from build123d import *

# Parameters (mm, degrees)
SKETCH2_R                      = 22.5
SKETCH2_R_2                    = 14.5
USB_CHARGE_DEVICE_RING_DEPTH   = 10
RING_START                     = 70.540362552
RING_COMPLETION_DEPTH          = 10
SKETCH4_W                      = 45
SKETCH4_H                      = 23.80144284
LINK_TO_UNIT_CHASSIS_DEPTH     = 8
SKETCH5_W                      = 100
SKETCH5_H                      = 166
SKETCH5_W_2                    = 94
SKETCH5_H_2                    = 160
CHASSIS_WALLS_DEPTH            = 55
SKETCH6_W                      = 19
SKETCH6_H                      = 19
SKETCH6_R                      = 1.75
DISPLAY_FRAME_MOUNT_TABS_DEPTH = 3
SKETCH7_W                      = 94
SKETCH7_H                      = 68
SKETCH7_R                      = 1
RPI_MOUNT_SURFACE_DEPTH        = 3
SKETCH8_R                      = 3
SKETCH8_R_2                    = 1
RPI_MOUNT_BOSSES_DEPTH         = 2
F_50MM_FAN_HOLES_REACH         = 246.023
SKETCH9_R                      = 1.75
SKETCH9_R_2                    = 25
RJ45_CUTOUT_REACH              = 246.023
SKETCH10_R                     = 1.75
SKETCH10_W                     = 14
SKETCH10_H                     = 17


# Read off the part's stored shape, not the designer's step: RING COMPLETION
with BuildPart() as part:
    # Sketch2 → USB CHARGE DEVICE RING (new body)
    with BuildSketch(Plane(origin=(0, 40.270181276, 69.75), x_dir=(1, 0, 0), z_dir=(0, 0.500000000000001, 0.866025403784438))):
        with Locations(Location((0, -117.602885683, 0), (0, 0, 270))):
            Circle(SKETCH2_R)
        with Locations(Location((0, -117.602885683, 0), (0, 0, 270))):
            Circle(SKETCH2_R_2, mode=Mode.SUBTRACT)
    extrude(amount=-USB_CHARGE_DEVICE_RING_DEPTH)

    # RING COMPLETION outline → RING COMPLETION (add)
    with BuildSketch(Plane(origin=(0, 0, 0), x_dir=(1, 0, 0), z_dir=(0, 0.500000000000001, 0.866025403784438)).offset(RING_START)):
        with BuildLine():
            Line((-22.5, -68.102885683), (-22.5, -117.602885683))
            ThreePointArc((-22.5, -117.602885683), (0, -95.102885683), (22.5, -117.602885683))
            Line((22.5, -117.602885683), (22.5, -68.102885683))
            Line((22.5, -68.102885683), (-22.5, -68.102885683))
        make_face()
    extrude(amount=RING_COMPLETION_DEPTH)

    # Sketch4 → LINK TO UNIT CHASSIS (add)
    with BuildSketch(Plane(origin=(0, -18.708647797, 0), x_dir=(1, 0, 0), z_dir=(0, 1, 0))):
        with Locations((0, -91.900721421)):
            Rectangle(SKETCH4_W, SKETCH4_H)
    extrude(amount=-LINK_TO_UNIT_CHASSIS_DEPTH)

    # Sketch5 → CHASSIS WALLS (add)
    with BuildSketch(Plane(origin=(0, -13.208647797, 0), x_dir=(-1, 0, 0), z_dir=(0, -1, 0))):
        Rectangle(SKETCH5_W, SKETCH5_H)
        Rectangle(SKETCH5_W_2, SKETCH5_H_2, mode=Mode.SUBTRACT)
    extrude(amount=CHASSIS_WALLS_DEPTH)

    # Sketch6 → DISPLAY FRAME MOUNT TABS (add)
    # profile 1 of 3: a face of its own
    with BuildSketch(Plane(origin=(0, -13.208647797, 0), x_dir=(1, 0, 0), z_dir=(0, 1, 0))):
        with Locations((-40.5, -73.5)):
            Rectangle(SKETCH6_W, SKETCH6_H)
        with Locations(Location((-36, -69, 0), (0, 0, 270))):
            Circle(SKETCH6_R, mode=Mode.SUBTRACT)
    # profile 2 of 3: a face of its own
    with BuildSketch(Plane(origin=(0, -13.208647797, 0), x_dir=(1, 0, 0), z_dir=(0, 1, 0))):
        with Locations((40.5, -73.5)):
            Rectangle(SKETCH6_W, SKETCH6_H)
        with Locations(Location((36, -69, 0), (0, 0, 270))):
            Circle(SKETCH6_R, mode=Mode.SUBTRACT)
    # profile 3 of 3: a face of its own
    with BuildSketch(Plane(origin=(0, -13.208647797, 0), x_dir=(1, 0, 0), z_dir=(0, 1, 0))):
        with Locations((40.5, 73.5)):
            Rectangle(SKETCH6_W, SKETCH6_H)
        with Locations(Location((36, 69, 0), (0, 0, 270))):
            Circle(SKETCH6_R, mode=Mode.SUBTRACT)
    extrude(amount=-DISPLAY_FRAME_MOUNT_TABS_DEPTH)

    # Sketch7 → RPI MOUNT SURFACE (add)
    with BuildSketch(Plane(origin=(0, -32.208647797, 0), x_dir=(-1, 0, 0), z_dir=(0, -1, 0))):
        with Locations((0, -30.000000001)):
            Rectangle(SKETCH7_W, SKETCH7_H)
        with Locations(Location((7, -1.000000001, 0), (0, 0, 90))):
            Circle(SKETCH7_R, mode=Mode.SUBTRACT)
        with Locations(Location((-42, -1.000000001, 0), (0, 0, 90))):
            Circle(SKETCH7_R, mode=Mode.SUBTRACT)
        with Locations(Location((7, -59.000000001, 0), (0, 0, 90))):
            Circle(SKETCH7_R, mode=Mode.SUBTRACT)
        with Locations(Location((-42, -59.000000001, 0), (0, 0, 90))):
            Circle(SKETCH7_R, mode=Mode.SUBTRACT)
    extrude(amount=RPI_MOUNT_SURFACE_DEPTH)

    # Sketch8 → RPI MOUNT BOSSES (add)
    # profile 1 of 4: a face of its own
    with BuildSketch(Plane.XZ.offset(35.208647797)):
        with Locations(Location((42, 59.000000001, 0), (0, 0, 270))):
            Circle(SKETCH8_R)
        with Locations(Location((42, 59.000000001, 0), (0, 0, 270))):
            Circle(SKETCH8_R_2, mode=Mode.SUBTRACT)
    # profile 2 of 4: a face of its own
    with BuildSketch(Plane.XZ.offset(35.208647797)):
        with Locations(Location((42, 1.000000001, 0), (0, 0, 270))):
            Circle(SKETCH8_R)
        with Locations(Location((42, 1.000000001, 0), (0, 0, 270))):
            Circle(SKETCH8_R_2, mode=Mode.SUBTRACT)
    # profile 3 of 4: a face of its own
    with BuildSketch(Plane.XZ.offset(35.208647797)):
        with Locations(Location((-7, 1.000000001, 0), (0, 0, 270))):
            Circle(SKETCH8_R)
        with Locations(Location((-7, 1.000000001, 0), (0, 0, 270))):
            Circle(SKETCH8_R_2, mode=Mode.SUBTRACT)
    # profile 4 of 4: a face of its own
    with BuildSketch(Plane.XZ.offset(35.208647797)):
        with Locations(Location((-7, 59.000000001, 0), (0, 0, 270))):
            Circle(SKETCH8_R)
        with Locations(Location((-7, 59.000000001, 0), (0, 0, 270))):
            Circle(SKETCH8_R_2, mode=Mode.SUBTRACT)
    extrude(amount=RPI_MOUNT_BOSSES_DEPTH)

    # Sketch9 → 50MM FAN HOLES (cut, up to next)
    with BuildSketch(Plane(origin=(0, 0, -83), x_dir=(-1, 0, 0), z_dir=(0, 0, -1)), mode=Mode.PRIVATE) as f_50mm_fan_holes_sk1:
        with Locations((-23, -20.708647797)):
            Circle(SKETCH9_R)
    f_50mm_fan_holes_tool1 = extrude(f_50mm_fan_holes_sk1.sketch, amount=-F_50MM_FAN_HOLES_REACH, mode=Mode.PRIVATE) & part.part
    # Sketch9 → 50MM FAN HOLES (cut, up to next)
    with BuildSketch(Plane(origin=(0, 0, -83), x_dir=(-1, 0, 0), z_dir=(0, 0, -1)), mode=Mode.PRIVATE) as f_50mm_fan_holes_sk2:
        with Locations((17, -20.708647797)):
            Circle(SKETCH9_R)
    f_50mm_fan_holes_tool2 = extrude(f_50mm_fan_holes_sk2.sketch, amount=-F_50MM_FAN_HOLES_REACH, mode=Mode.PRIVATE) & part.part
    # Sketch9 → 50MM FAN HOLES (cut, up to next)
    with BuildSketch(Plane(origin=(0, 0, -83), x_dir=(-1, 0, 0), z_dir=(0, 0, -1)), mode=Mode.PRIVATE) as f_50mm_fan_holes_sk3:
        with Locations((17, -60.708647797)):
            Circle(SKETCH9_R)
    f_50mm_fan_holes_tool3 = extrude(f_50mm_fan_holes_sk3.sketch, amount=-F_50MM_FAN_HOLES_REACH, mode=Mode.PRIVATE) & part.part
    # Sketch9 → 50MM FAN HOLES (cut, up to next)
    with BuildSketch(Plane(origin=(0, 0, -83), x_dir=(-1, 0, 0), z_dir=(0, 0, -1)), mode=Mode.PRIVATE) as f_50mm_fan_holes_sk4:
        with Locations((-23, -60.708647797)):
            Circle(SKETCH9_R)
    f_50mm_fan_holes_tool4 = extrude(f_50mm_fan_holes_sk4.sketch, amount=-F_50MM_FAN_HOLES_REACH, mode=Mode.PRIVATE) & part.part
    # Sketch9 → 50MM FAN HOLES (cut, up to next)
    with BuildSketch(Plane(origin=(0, 0, -83), x_dir=(-1, 0, 0), z_dir=(0, 0, -1)), mode=Mode.PRIVATE) as f_50mm_fan_holes_sk5:
        with Locations((-3, -40.708647797)):
            Circle(SKETCH9_R_2)
    f_50mm_fan_holes_tool5 = extrude(f_50mm_fan_holes_sk5.sketch, amount=-F_50MM_FAN_HOLES_REACH, mode=Mode.PRIVATE) & part.part
    add(f_50mm_fan_holes_tool1.solids().sort_by_distance((23, -20.708648, -83))[0], mode=Mode.SUBTRACT)
    add(f_50mm_fan_holes_tool2.solids().sort_by_distance((-17, -20.708648, -83))[0], mode=Mode.SUBTRACT)
    add(f_50mm_fan_holes_tool3.solids().sort_by_distance((-17, -60.708648, -83))[0], mode=Mode.SUBTRACT)
    add(f_50mm_fan_holes_tool4.solids().sort_by_distance((23, -60.708648, -83))[0], mode=Mode.SUBTRACT)
    add(f_50mm_fan_holes_tool5.solids().sort_by_distance((3, -40.708648, -83))[0], mode=Mode.SUBTRACT)

    # Sketch10 → RJ45 CUTOUT (cut, up to next)
    with BuildSketch(Plane(origin=(0, 0, -83), x_dir=(-1, 0, 0), z_dir=(0, 0, -1)), mode=Mode.PRIVATE) as rj45_cutout_sk1:
        with Locations((35, -29.708647797)):
            Circle(SKETCH10_R)
    rj45_cutout_tool1 = extrude(rj45_cutout_sk1.sketch, amount=-RJ45_CUTOUT_REACH, mode=Mode.PRIVATE) & part.part
    # Sketch10 → RJ45 CUTOUT (cut, up to next)
    with BuildSketch(Plane(origin=(0, 0, -83), x_dir=(-1, 0, 0), z_dir=(0, 0, -1)), mode=Mode.PRIVATE) as rj45_cutout_sk2:
        with Locations((35, -56.708647797)):
            Circle(SKETCH10_R)
    rj45_cutout_tool2 = extrude(rj45_cutout_sk2.sketch, amount=-RJ45_CUTOUT_REACH, mode=Mode.PRIVATE) & part.part
    # Sketch10 → RJ45 CUTOUT (cut, up to next)
    with BuildSketch(Plane(origin=(0, 0, -83), x_dir=(-1, 0, 0), z_dir=(0, 0, -1)), mode=Mode.PRIVATE) as rj45_cutout_sk3:
        with Locations((33.5, -43.208647797)):
            Rectangle(SKETCH10_W, SKETCH10_H)
    rj45_cutout_tool3 = extrude(rj45_cutout_sk3.sketch, amount=-RJ45_CUTOUT_REACH, mode=Mode.PRIVATE) & part.part
    add(rj45_cutout_tool1.solids().sort_by_distance((-35, -29.708648, -83))[0], mode=Mode.SUBTRACT)
    add(rj45_cutout_tool2.solids().sort_by_distance((-35, -56.708648, -83))[0], mode=Mode.SUBTRACT)
    add(rj45_cutout_tool3.solids().sort_by_distance((-33.5, -43.208648, -83))[0], mode=Mode.SUBTRACT)


solid = part.part
Geometry check sheet. Reference: the model listing, model coordinates, mm. A direction names the side the tool comes from. Coordinates: 2 decimals unless noted, no trailing zeros. Loops run counter-clockwise (first coordinate to the right, second up) from the corner with the lowest first, then second, coordinate; pieces in that order, holes last. Notation, with made-up numbers: (-30, -1) - (-2, -1) arc R36 ccw to (-2, 36) - close; hole circle Ø2 at (89, 78.25). An arc over 180 degrees is marked (long way). Use one line per item in the form item = value. Start each with the question number.
Item 1: Gauge pin test, flat ends, axial feed: pin 1 (15.5 mm diameter, centred on x = 10.5, z = 93, fed in from -Y); pin 2 (17.5 mm diameter, centred on x = -40, z = 73, fed in from -Y); pin 3 (1 mm diameter, centred on x = 7, y = -31, fed in from -Z); pin 4 (4.5 mm diameter, centred on x = -35, y = -56.71, fed in from -Z). Record the tip position at first contact, or that the pin passes through.
Item 2: Tool access check on faces 1 (the face through (-47, -40, 1)), 2 (the face through (-20, -53, -80)), 3 (the face through (-6, -37.209, 2)), 4 (the face through (-22.5, -37, 108)), 5 (the face through (22.5, -39, 108)). Record the directions out of +Z, -Z, +X, -X, +Y, -Y that give a thin tool (end or side, any length) a straight path to the whole face; none if there is none.
Item 3: Mould release check, pull along Z, two halves, no side actions. Record for faces 6 (the face through (-22, -46, -83)), 7 (the face through (1, -40, 80)), 8 (the face through (48, -13.209, 0)): +Z half, -Z half, draft (parallel to the pull), parting line (faces both ways), or undercut.
Item 4: Thickness scan on probe 1 along X at (y, z) = (-34, 59); probe 2 along Z at (x, y) = (45.5, -22); probe 3 along X at (y, z) = (-38, -24). Record the ranges inside material, lowest first.
Item 5: Section check A-A, the plane z = -17.5. Enter the section's corners in (x, y), and give its area (3 significant figures).
Item 6: Section check B-B, the plane z = 35. Enter the section's corners in (x, y), and give its area (3 significant figures).
Computed:
q1.pin_1 = -33.42
q1.pin_2 = -68.21
q1.pin_3 = 80
q1.pin_4 = -83
q2.face_1 = none
q2.face_2 = -Y
q2.face_3 = -Z, -Y
q2.face_4 = +Z, -X, +Y, -Y
q2.face_5 = +Z, +X, +Y, -Y
q3.face_6 = -Z half
q3.face_7 = undercut
q3.face_8 = draft
q4.probe_1 = -50 to -8, -6 to 41, 43 to 50
q4.probe_2 = -83 to -80, 80 to 83
q4.probe_3 = -50 to -47, 47 to 50
q5.outline = (-50, -68.21) - (-47, -68.21) - (-47, -13.21) - (-50, -13.21) - close; (47, -68.21) - (50, -68.21) - (50, -13.21) - (47, -13.21) - close
q5.area = 330 mm2
q6.outline = (-50, -68.21) - (-47, -68.21) - (-47, -35.21) - (47, -35.21) - (47, -68.21) - (50, -68.21) - (50, -13.21) - (47, -13.21) - (47, -32.21) - (-47, -32.21) - (-47, -13.21) - (-50, -13.21) - close
q6.area = 612 mm2
